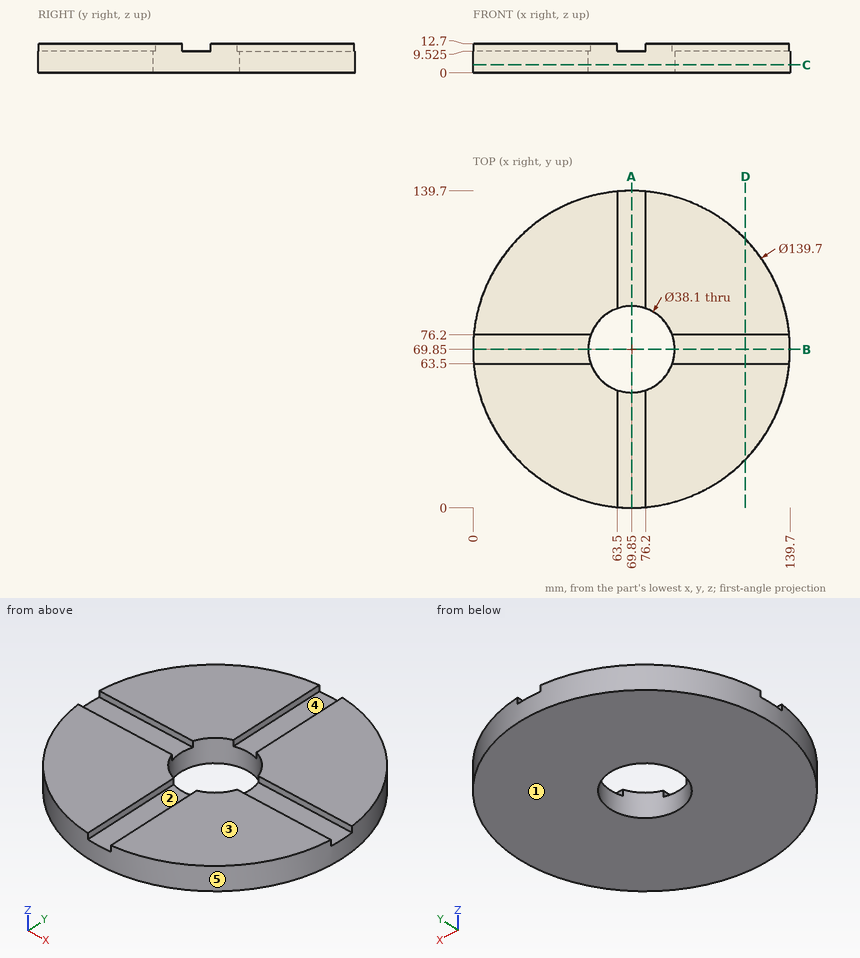
The drawing under review shows one solid part. Ordinate dimensions are in mm from its lowest x, y, z. A direction names the side the tool comes from. Coordinates: 2 decimals unless noted, no trailing zeros. Order: outer loops, then holes, each group sorted by start corner. A loop starts at its lowest first (then second) coordinate and runs counter-clockwise, first axis right, second up. Notation, with made-up numbers: (7, -2.75) -> (13, -2.75) arc R10 ccw to (13, 14.25) -> close; hole circle Ø1 at (-22, 50.25). An arc over 180 degrees is marked (long way). Answer in a Markdown table with one row per item. Add a question column.
Item 1: Mouldability with a two-part tool opening along X and no side actions: class the marked faces 3, 4 and 5 as +X half, -X half, draft (parallel to the pull), parting line (faces both ways), or undercut.
Item 2: Clearance check with flat-ended pins moving along their axes: pin 1 (6 mm diameter, centred on y = 95, z = 2, fed in from +X) (3 decimals); pin 2 (1.5 mm diameter, centred on x = 25, z = 7.5, fed in from -Y); pin 3 (3 mm diameter, centred on y = 86, z = 6.5, fed in from -X). State where each tip first meets the part, or that it passes through.
Item 3: Machinability: for the marked faces 1 and 2, which of the approach directions +Z, -Z, +X, -X, +Y, -Y give a long, thin tool a straight path to every point of the face, cutting with its end or side? Answer none if there is none.
Item 4: We need section D-D on x = 120. Write out the cut boundary in (y, z) (3 decimals).
Item 5: We need section A-A on x = 69.85. Write out the cut boundary in (y, z) (3 decimals).
Item 6: We need section C-C on z = 3.5. Write out the cut boundary in (x, y), plus the area to 3 significant figures.
Item 7: To check wall thickness, follow probe 1 along X at (y, z) = (69.85, 3); probe 2 along Z at (x, y) = (73, 29.5) (3 decimals). State the ranges of each line that lie inside material, in increasing order.
Final values:
| question | item | result |
|---|---|---|
| 1 | face 3 | draft |
| 1 | face 4 | undercut |
| 1 | face 5 | parting line |
| 2 | pin 1 | stops at x = 136.095 |
| 2 | pin 2 | stops at y = 15.68 |
| 2 | pin 3 | stops at x = 1.55 |
| 3 | face 1 | -Z, +X, -X, +Y, -Y |
| 3 | face 2 | +Z, +Y, -Y |
| 4 | outline | (21.229, 0) -> (118.471, 0) -> (118.471, 12.7) -> (76.2, 12.7) -> (76.2, 9.525) -> (63.5, 9.525) -> (63.5, 12.7) -> (21.229, 12.7) -> close |
| 5 | outline | (0, 0) -> (50.8, 0) -> (50.8, 9.525) -> (0, 9.525) -> close; (88.9, 0) -> (139.7, 0) -> (139.7, 9.525) -> (88.9, 9.525) -> close |
| 6 | outline | circle Ø139.7 at (69.85, 69.85); hole circle Ø38.1 at (69.85, 69.85) |
| 6 | area | 14,200 mm2 |
| 7 | probe 1 | x = 0 to 50.8, 88.9 to 139.7 |
| 7 | probe 2 | z = 0 to 9.525 |
